from build123d import *

# Parameters (mm, degrees)
F1_DEPTH = 320
F2_R     = 5
F4_D     = 17.5
F4_DEPTH = 20
F4_TIP   = 5.2575304165
F5_R     = 5
F6_R     = 5


with BuildPart() as f1:
    # F0 (on Front) → F1 (new body)
    with BuildSketch(Plane.XZ):
        Polygon((5, -45), (5, 45), (-5, 45), (-5, -45), (-5, -55), (295, -55), (295, -45), align=None)
    extrude(amount=-F1_DEPTH)

    # F2
    f2_edges = [f1.edges().sort_by_distance(p)[0] for p in [
        (0, 0, 45),
        (0, 320, 45),
        (295, 320, -50),
        (295, 0, -50),
    ]]
    fillet(f2_edges, radius=F2_R)

    # F4
    with Locations(Plane.YZ.offset(5)):
        with Locations((20, -25), (20, 25), (300, 25), (300, -25)):
            Hole(F4_D / 2, depth=F4_DEPTH)
            with Locations((0, 0, -(F4_DEPTH + F4_TIP / 2))):  # 118° drill point
                Cone(0, F4_D / 2, F4_TIP, mode=Mode.SUBTRACT)

    # F5
    f5_edges = [f1.edges().sort_by_distance(p)[0] for p in [
        (-5, 160, -55),
    ]]
    fillet(f5_edges, radius=F5_R)

    # F6
    f6_edges = [f1.edges().sort_by_distance(p)[0] for p in [
        (5, 160, -45),
    ]]
    fillet(f6_edges, radius=F6_R)


solid = f1.part
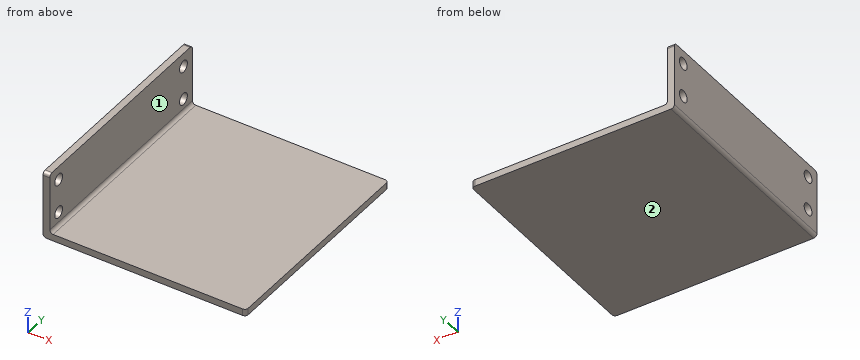
Work out the finished part from the listing and answer in its coordinate system (mm). Face numbers are marked on the shaded views. A direction names the side the tool comes from. Coordinates: 2 decimals unless noted, no trailing zeros. Write each loop counter-clockwise with the first axis right and the second up, starting at its lowest first coordinate (ties: lowest second). Pieces come first, ordered by that corner, then holes. Notation, with made-up numbers: (52.5, 66) - (57.5, 66) arc R18 cw to (57.5, 93) - close; hole circle Ø9 at (21, 83.25). An arc over 180 degrees is marked (long way). One line per question, with ' | ' between items.
1) Find section C-C, the plane y = 267. Determine the outline of the cut face in (x, z).
Checks:
outline: (-5, -50) arc R5 ccw to (0, -55) - (295, -55) - (295, -45) - (10, -45) arc R5 cw to (5, -40) - (5, 45) - (-5, 45) - close
2) Flat-ended cylindrical pins translate along their axes: P1, Ø4, axis at y = 147, z = 31.5, coming from the +X side; P2, Ø4, axis at x = 169, y = 39.5, coming from the +Z side. Find the tip coordinate at first contact, or state that the pin passes through.
Checks:
P1: x = 5 | P2: z = -45
3) Find section B-B, the plane z = -25. Determine the outline of the cut face in (x, y), and give its area (3 significant figures).
Checks:
outline: (-5, 0) - (5, 0) - (5, 11.25) - (-5, 11.25) - close; (-5, 28.75) - (5, 28.75) - (5, 291.25) - (-5, 291.25) - close; (-5, 308.75) - (5, 308.75) - (5, 320) - (-5, 320) - close | area: 2,850 mm2
4) Find section D-D, the plane x = 109. Determine the outline of the cut face in (y, z), and give its area (3 significant figures).
Checks:
outline: (0, -55) - (320, -55) - (320, -45) - (0, -45) - close | area: 3,200 mm2
5) Find section A-A, the plane y = 20. Determine the outline of the cut face in (x, z), and give its area (3 significant figures).
Checks:
outline: (-5, -50) arc R5 ccw to (0, -55) - (295, -55) - (295, -45) - (10, -45) arc R5 cw to (5, -40) - (5, -33.75) - (-5, -33.75) - close; (-5, -16.25) - (5, -16.25) - (5, 16.25) - (-5, 16.25) - close; (-5, 33.75) - (5, 33.75) - (5, 45) - (-5, 45) - close | area: 3,550 mm2
6) For the marked faces 1 and 2, determine the directions among +Z, -Z, +X, -X, +Y, -Y from which every point of the face is accessible in a straight line to the end or side of a thin tool.
Checks:
face 1: +Z, +X, +Y, -Y | face 2: -Z, +X, -X, +Y, -Y
7) Consider probe 1 along Z at (x, y) = (2, 300); probe 2 along Z at (x, y) = (-1.75, 300); probe 3 along Z at (x, y) = (167, 202). Determine where each line is inside the solid, lowest interval first. Write a range as [from, to].
Checks:
probe 1: [-55, -33.75], [-16.25, 16.25], [33.75, 45] | probe 2: [-54.68, -33.75], [-16.25, 16.25], [33.75, 45] | probe 3: [-55, -45]
